```python
from build123d import *

# Parameters (mm, degrees)
SKIZZE1_R                       = 2.5
SKIZZE1_R_2                     = 1.5
AUFSATZ_LINEAR_AUSTRAGEN1_DEPTH = 4


with BuildPart() as part:
    # Skizze1 → Aufsatz-Linear austragen1 (new body)
    # profile 1 of 3: a face of its own
    with BuildSketch(Plane.XY):
        with Locations((0, 30)):
            Circle(SKIZZE1_R)
        with Locations((0, 30)):
            Circle(SKIZZE1_R_2, mode=Mode.SUBTRACT)
    # profile 2 of 3: a face of its own
    with BuildSketch(Plane.XY):
        with BuildLine():
            ThreePointArc((2.5, 30), (0, 27.5), (-2.5, 30))
            Line((-2.5, 30), (-2.5, 0))
            ThreePointArc((-2.5, 0), (0, 2.5), (2.5, 0))
            Line((2.5, 0), (2.5, 30))
        make_face()
    # profile 3 of 3: a face of its own
    with BuildSketch(Plane.XY):
        Circle(SKIZZE1_R)
        Circle(SKIZZE1_R_2, mode=Mode.SUBTRACT)
    extrude(amount=AUFSATZ_LINEAR_AUSTRAGEN1_DEPTH)


solid = part.part
```
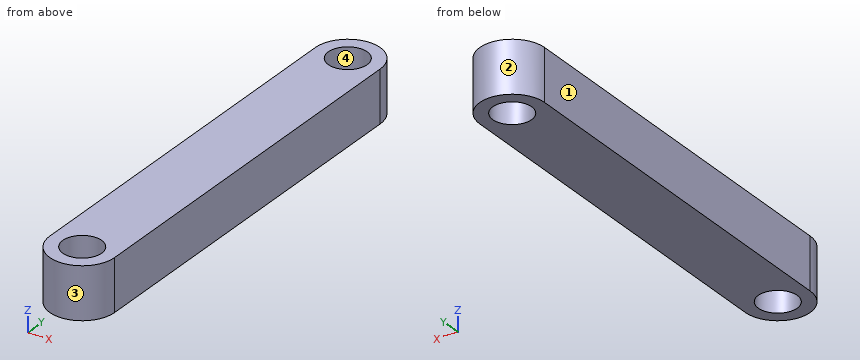
Can you work these out from the model? Positions are in its coordinate system, mm. Face numbers are marked on the shaded views. Round coordinates to 2 decimals unless told otherwise and drop trailing zeros. Loops run counter-clockwise (first coordinate to the right, second up) from the corner with the lowest first, then second, coordinate; pieces in that order, holes last. Notation, with made-up numbers: M 25.5,81 L 34.5,81 A35 cw 34.5,120 Z; hole C 15.25,67.5 d7. An arc over 180 degrees is marked long. Answer as a JSON object with one key per item and string values. Group by question number.
Q1. Please list where these lines run through material, in increasing order: L1, parallel to Y at x = 0, z = 3.1; L2, parallel to Y at x = -0.5, z = 2.85; L3, parallel to Y at x = 1.95, z = 3.7.
Q2. Imagine slicing it at B-B, the plane x = 1. Please give me the cut outline in (y, z), then the cut area to 3 significant figures.
Q3. Imagine slicing it at A-A, the plane z = 1. Please give me the cut outline in (x, y).
Q4. We'd pull the mould along Y, two halves only. Please class the marked faces 1, 2, 3 and 4: +Y half, -Y half, draft (parallel to the pull), parting line (faces both ways), or undercut.
Q5. Will these pins go through, and if not, where does the flat tip stop? pin 1 (1.8 mm diameter, centred on x = 0, y = 30, fed in from -Z); pin 2 (2 mm diameter, centred on x = 1, z = 3, fed in from -Y).
Q6. Imagine slicing it at D-D, the plane x = -1.85. Please give me the cut outline in (y, z).
Q7. Imagine slicing it at C-C, the plane x = -0.25. Please give me the cut outline in (y, z), then the cut area to 3 significant figures.
Findings:
{
 "1": {"L1": "y = -2.5 to -1.5, 1.5 to 28.5, 31.5 to 32.5", "L2": "y = -2.45 to -1.41, 1.41 to 28.59, 31.41 to 32.45", "L3": "y = -1.56 to 31.56"},
 "2": {"outline": "M -2.29,0 L -1.12,0 L -1.12,4 L -2.29,4 Z; M 1.12,0 L 28.88,0 L 28.88,4 L 1.12,4 Z; M 31.12,0 L 32.29,0 L 32.29,4 L 31.12,4 Z", "area": "120 mm2"},
 "3": {"outline": "M -2.5,0 A2.5 ccw 2.5,0 L 2.5,30 A2.5 ccw -2.5,30 Z; hole C 0,0 d3; hole C 0,30 d3"},
 "4": {"face 1": "draft", "face 2": "+Y half", "face 3": "-Y half", "face 4": "undercut"},
 "5": {"pin 1": "passes through", "pin 2": "stops at y = -2.5"},
 "6": {"outline": "M -1.68,0 L 31.68,0 L 31.68,4 L -1.68,4 Z"},
 "7": {"outline": "M -2.49,0 L -1.48,0 L -1.48,4 L -2.49,4 Z; M 1.48,0 L 28.52,0 L 28.52,4 L 1.48,4 Z; M 31.48,0 L 32.49,0 L 32.49,4 L 31.48,4 Z", "area": "116 mm2"}
}
